Could you check a few things on this model? Use its own coordinates, in mm. A direction names the side the tool comes from. Round coordinates to 2 decimals unless told otherwise and drop trailing zeros. Write each loop counter-clockwise with the first axis right and the second up, starting at its lowest first coordinate (ties: lowest second). Pieces come first, ordered by that corner, then holes. Notation, with made-up numbers: M 29,-37.5 L 79,-37.5 A25 ccw 79,-11.5 Z; hole C -28,73.5 d2. An arc over 180 degrees is marked long. One line per item, written item: value. Start each with the question number.
(1) Thinking about a two-plate mould opening in X: for faces 1 (the face through (109, 25.7, -83)), 2 (the face through (5.98, 0.99, -8.1)), 3 (the face through (164.17, 15.99, -82.6)), 4 (the face through (100.273, 15.988, -82.605)), which applies, released by +X, released by -X, zero draft, split by the parting line, or undercut?
(2) I'm going to push flat-ended pins straight in: pin 1 Ø6 at (y, z) = (8.5, -72) entering from +X; pin 2 Ø4 at (x, z) = (125.5, -9) entering from +Y; pin 3 Ø2 at (x, z) = (5, -85.5) entering from -Y; pin 4 Ø5 at (x, z) = (6, -36.5) entering from +Y. Where does each tip first touch, or does it pass through?
(3) I want a section at A-A on z = -11. Please give me the cut outline in (x, y), and give its area (3 significant figures).
(4) I want a section at C-C on y = 20.78. Count the separate pieces of the cut face and the enclosed holes in it, and give its area (3 significant figures).
(5) I want a section at D-D on z = -63. Please give me the cut outline in (x, y), and give its area (3 significant figures).
(6) I want a section at B-B on x = 108.2. Please give me the cut outline in (y, z) (3 decimals), and give its area (3 significant figures).
(7) Which directions (+Z, -Z, +X, -X, +Y, -Y) give clear straight access to the entire face, cutting with the end or side of a thin tool? Please do faces 5 (the face through (171.827, 0.986, -84.295)), 6 (the face through (112.46, 13, -13)), 7 (the face through (159, 14, -15)).
(8) If I drill on L1, parallel to Z at x = 175, y = 4.7 (3 decimals); L2, parallel to Z at x = 175, y = 1.6; L3, parallel to Y at x = 157.7, z = -82.75 (3 decimals), over which ranges is the centre line in solid material (lowest first)?
```python
from build123d import *

# Parameters (mm, degrees)
SKIZZE2_W                       = 180
SKIZZE2_H                       = 90
AUFSATZ_LINEAR_AUSTRAGEN1_DEPTH = 6
SKIZZE3_W                       = 10
SKIZZE3_H                       = 90
SCHNITT_LINEAR_AUSTRAGEN1_DEPTH = 3
SKIZZE4_R                       = 2.125
AUFSATZ_LINEAR_AUSTRAGEN2_DEPTH = 15
SKIZZE5_R                       = 2.1
AUFSATZ_LINEAR_AUSTRAGEN3_DEPTH = 15
VERRUNDUNG1_R                   = 5
SCHNITT_LINEAR_AUSTRAGEN2_DEPTH = 10
SKIZZE7_R                       = 0.975
SCHNITT_LINEAR_AUSTRAGEN3_DEPTH = 10
SKIZZE8_R                       = 3.25
SCHNITT_LINEAR_AUSTRAGEN4_DEPTH = 2


with BuildPart() as part:
    # Skizze2 → Aufsatz-Linear austragen1 (new body)
    with BuildSketch(Plane(origin=(0, 0, 0), x_dir=(1, 0, 0), z_dir=(0, 1, 0))):
        with Locations((90, 45)):
            Rectangle(SKIZZE2_W, SKIZZE2_H)
    extrude(amount=AUFSATZ_LINEAR_AUSTRAGEN1_DEPTH)

    # Skizze3 → Schnitt-Linear austragen1 (cut)
    with BuildSketch(Plane(origin=(0, 6, 0), x_dir=(1, 0, 0), z_dir=(0, 1, 0))):
        with Locations((5, 45)):
            Rectangle(SKIZZE3_W, SKIZZE3_H)
    extrude(amount=-SCHNITT_LINEAR_AUSTRAGEN1_DEPTH, mode=Mode.SUBTRACT)

    # Skizze4 → Aufsatz-Linear austragen2 (add)
    # profile 1 of 2: a face of its own
    with BuildSketch(Plane(origin=(0, 0, -90), x_dir=(-1, 0, 0), z_dir=(0, 0, -1))):
        Polygon((-160, 0), (-152.94, 0), (-152.94, 25.7), (-160, 25.7), (-168.464332067, 6), (-160, 6), align=None)
        with Locations((-157.7, 20.78)):
            Circle(SKIZZE4_R, mode=Mode.SUBTRACT)
    # profile 2 of 2: a face of its own
    with BuildSketch(Plane(origin=(0, 0, -90), x_dir=(-1, 0, 0), z_dir=(0, 0, -1))):
        Polygon((-105.4, 25.7), (-95, 6), (-105.4, 6), (-105.4, 0), (-112.46, 0), (-112.46, 25.7), align=None)
        with Locations((-108.2, 20.78)):
            Circle(SKIZZE4_R, mode=Mode.SUBTRACT)
    extrude(amount=-AUFSATZ_LINEAR_AUSTRAGEN2_DEPTH)

    # Skizze5 → Aufsatz-Linear austragen3 (add)
    # profile 1 of 2: a face of its own
    with BuildSketch(Plane.XY):
        Polygon((105.4, 25.7), (95, 6), (105.4, 6), (112.46, 6), (112.46, 25.7), align=None)
        with Locations((108.2, 20.78)):
            Circle(SKIZZE5_R, mode=Mode.SUBTRACT)
    # profile 2 of 2: a face of its own
    with BuildSketch(Plane.XY):
        Polygon((160, 25.7), (152.94, 25.7), (152.94, 6), (160, 6), (168.464332067, 6), align=None)
        with Locations((157.7, 20.78)):
            Circle(SKIZZE5_R, mode=Mode.SUBTRACT)
    extrude(amount=-AUFSATZ_LINEAR_AUSTRAGEN3_DEPTH)

    # Verrundung1
    verrundung1_edges = [part.edges().sort_by_distance(p)[0] for p in [
        (180, 0, -45),
    ]]
    fillet(verrundung1_edges, radius=VERRUNDUNG1_R)

    # Skizze6 → Schnitt-Linear austragen2 (cut)
    with BuildSketch(Plane(origin=(0, 0, 0), x_dir=(-1, 0, 0), z_dir=(0, -1, 0))):
        with BuildLine():
            Line((-117.46, 8), (-147.94, 8))
            ThreePointArc((-147.94, 8), (-151.475533906, 9.464466094), (-152.94, 13))
            Line((-152.94, 13), (-152.94, 32.5))
            ThreePointArc((-152.94, 32.5), (-151.475533906, 36.035533906), (-147.94, 37.5))
            Line((-147.94, 37.5), (-132.970987797, 37.5))
            Line((-132.970987797, 37.5), (-118.04, 37.5))
            ThreePointArc((-118.04, 37.5), (-114.094344161, 35.865655839), (-112.46, 31.92))
            Line((-112.46, 31.92), (-112.46, 13))
            ThreePointArc((-112.46, 13), (-113.924466094, 9.464466094), (-117.46, 8))
        make_face()
        with BuildLine():
            Line((-117.46, 82), (-147.94, 82))
            ThreePointArc((-147.94, 82), (-151.475533906, 80.535533906), (-152.94, 77))
            Line((-152.94, 77), (-152.94, 57.5))
            ThreePointArc((-152.94, 57.5), (-151.475533906, 53.964466094), (-147.94, 52.5))
            Line((-147.94, 52.5), (-117.46, 52.5))
            ThreePointArc((-117.46, 52.5), (-113.924466094, 53.964466094), (-112.46, 57.5))
            Line((-112.46, 57.5), (-112.46, 77))
            ThreePointArc((-112.46, 77), (-113.924466094, 80.535533906), (-117.46, 82))
        make_face()
    extrude(amount=-SCHNITT_LINEAR_AUSTRAGEN2_DEPTH, mode=Mode.SUBTRACT)

    # Skizze7 → Schnitt-Linear austragen3 (cut)
    with BuildSketch(Plane.XZ):
        with Locations(Location((5, -5, 0), (0, 0, 270))):
            Circle(SKIZZE7_R)
        with Locations(Location((5, -85, 0), (0, 0, 270))):
            Circle(SKIZZE7_R)
        with Locations(Location((175, -85, 0), (0, 0, 270))):
            Circle(SKIZZE7_R)
        with Locations(Location((175, -5, 0), (0, 0, 270))):
            Circle(SKIZZE7_R)
    extrude(amount=-SCHNITT_LINEAR_AUSTRAGEN3_DEPTH, mode=Mode.SUBTRACT)

    # Skizze8 → Schnitt-Linear austragen4 (cut)
    with BuildSketch(Plane.XZ):
        with Locations(Location((5, -5, 0), (0, 0, 270))):
            Circle(SKIZZE8_R)
        with Locations(Location((5, -85, 0), (0, 0, 270))):
            Circle(SKIZZE8_R)
        with Locations(Location((175, -85, 0), (0, 0, 270))):
            Circle(SKIZZE8_R)
        with Locations(Location((175, -5, 0), (0, 0, 270))):
            Circle(SKIZZE8_R)
    extrude(amount=-SCHNITT_LINEAR_AUSTRAGEN4_DEPTH, mode=Mode.SUBTRACT)


solid = part.part
```
Found:
1. face 1: zero draft
1. face 2: undercut
1. face 3: released by +X
1. face 4: released by -X
2. pin 1: stops at x = 180
2. pin 2: stops at y = 6
2. pin 3: stops at y = 2
2. pin 4: stops at y = 3
3. outline: M 0,0 L 112.88,0 L 112.88,6 L 112.46,6 L 112.46,25.7 L 105.4,25.7 L 95,6 L 10,6 L 10,3 L 0,3 Z; M 152.52,0 L 175,0 A5 ccw 180,5 L 180,6 L 168.46,6 L 160,25.7 L 152.94,25.7 L 152.94,6 L 152.52,6 Z; hole C 108.2,20.78 d4.2; hole C 157.7,20.78 d4.2
3. area: 1,240 mm²
4. separate pieces: 8
4. enclosed holes: 0
4. area: 311 mm²
5. outline: M 0,0 L 112.46,0 L 112.46,6 L 10,6 L 10,3 L 0,3 Z; M 152.94,0 L 175,0 A5 ccw 180,5 L 180,6 L 152.94,6 Z
5. area: 802 mm²
6. outline: M 0,-90 L 18.655,-90 L 18.655,-75 L 6,-75 L 6,-15 L 18.68,-15 L 18.68,0 L 0,0 Z; M 22.88,-15 L 25.7,-15 L 25.7,0 L 22.88,0 Z; M 22.905,-90 L 25.7,-90 L 25.7,-75 L 22.905,-75 Z
6. area: 1,000 mm²
7. face 5: -Y
7. face 6: +Y
7. face 7: +X, -X, +Y
8. L1: z = -90 to -85.975, -84.025 to -5.975, -4.025 to 0
8. L2: z = -90 to -88.25, -81.75 to -8.25, -1.75 to 0
8. L3: y = 0 to 18.655, 22.905 to 25.7
